Build history of the part. All positions in model axes, mm. Face numbers are marked on the shaded views. A direction names the side the tool comes from. Give positions to 0.01 mm unless a question says otherwise; leave off trailing zeros. Loops run counter-clockwise (first coordinate to the right, second up) from the corner with the lowest first, then second, coordinate; pieces in that order, holes last. Notation, with made-up numbers: (-18.75, 88.5) -> (-12.75, 88.5) arc R27 cw to (-12.75, 127.5) -> close; hole circle Ø10 at (49.5, 2). An arc over 180 degrees is marked (long way). Answer in a Markdown table with one row per item. Add a question column.
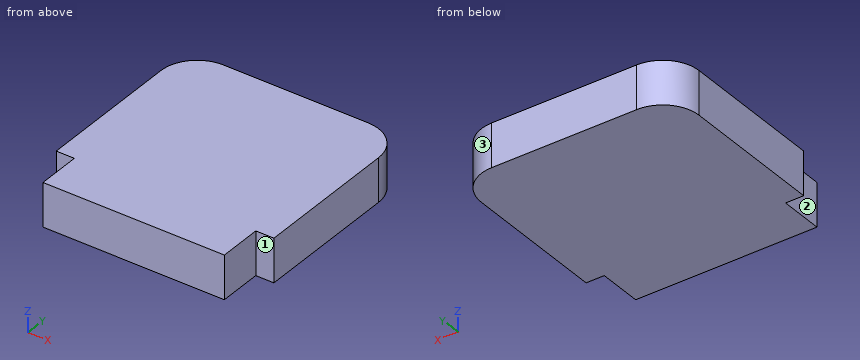
from build123d import *

# Parameters (mm, degrees)
ESBO_O1_W                = 30
ESBO_O1_H                = 25
ESBO_O1_W_2              = 25
ESBO_O1_H_2              = 6
RESSALTO_EXTRUS_O1_DEPTH = 6
FILETE1_R                = 5


with BuildPart() as part:
    # Esboço1 → Ressalto-extrusão1 (new body)
    with BuildSketch(Plane.XY):
        Rectangle(ESBO_O1_W, ESBO_O1_H)
        with Locations((0, -15.5)):
            Rectangle(ESBO_O1_W_2, ESBO_O1_H_2)
    extrude(amount=RESSALTO_EXTRUS_O1_DEPTH)

    # Filete1
    filete1_edges = [part.edges().sort_by_distance(p)[0] for p in [
        (-15, 12.5, 3),
        (15, 12.5, 3),
    ]]
    fillet(filete1_edges, radius=FILETE1_R)


solid = part.part
(1) Wall check: line 1 along X through (y, z) = (-16.5, 3.35); line 2 along X through (y, z) = (10, 3.9); line 3 along Y through (x, z) = (13.5, 5.5). Give the ranges that are in metal, low to high. Write a range as from..to.
(2) Flat gauge pins, fed straight in: pin 1 Ø1.2 at (x, z) = (13.5, 1.5) entering from -Y; pin 2 Ø3 at (x, y) = (11.5, 3.5) entering from -Z; pin 3 Ø1.8 at (y, z) = (-14.5, 1.5) entering from +X. Where does each tip first touch, or does it go through?
(3) Saw through at A-A, the plane z = 3.3. List the corners of the cut face in (x, y).
(4) Saw through at B-B, the plane y = -14. List the corners of the cut face in (x, z).
(5) 3-axis set-ups, long thin cutter, end or side, ignore diameter. For the marked faces 1, 2 and 3: which of +Z, -Z, +X, -X, +Y, -Y reach the whole face in a straight line?
Worked answers:
| question | item | result |
|---|---|---|
| 1 | line 1 | -12.5..12.5 |
| 1 | line 2 | -14.33..14.33 |
| 1 | line 3 | -12.5..11.07 |
| 2 | pin 1 | y = -12.5 |
| 2 | pin 2 | z = 0 |
| 2 | pin 3 | x = 12.5 |
| 3 | outline | (-15, -12.5) -> (-12.5, -12.5) -> (-12.5, -18.5) -> (12.5, -18.5) -> (12.5, -12.5) -> (15, -12.5) -> (15, 7.5) arc R5 ccw to (10, 12.5) -> (-10, 12.5) arc R5 ccw to (-15, 7.5) -> close |
| 4 | outline | (-12.5, 0) -> (12.5, 0) -> (12.5, 6) -> (-12.5, 6) -> close |
| 5 | face 1 | +Z, -Z, +X, -Y |
| 5 | face 2 | +Z, -Z, -X, -Y |
| 5 | face 3 | +Z, -Z, +X, +Y |
